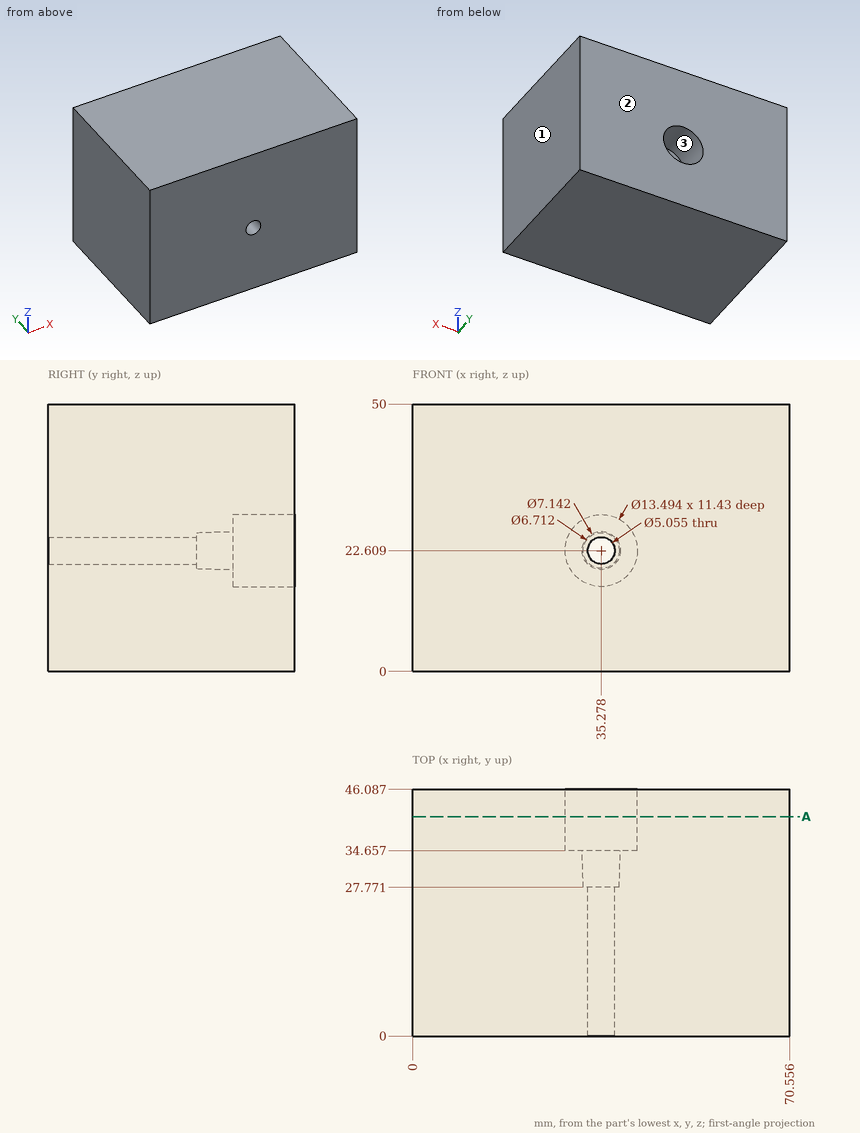
Job drawing, mm, ordinate dimensions from the low corner. One solid piece. Give positions to 0.01 mm unless a question says otherwise; leave off trailing zeros. Write each loop counter-clockwise with the first axis right and the second up, starting at its lowest first coordinate (ties: lowest second). Pieces come first, ordered by that corner, then holes. Notation, with made-up numbers: M 8,79.25 L 22,79.25 A7 ccw 22,90.25 Z; hole C 13.25,2.5 d6. An arc over 180 degrees is marked long. One line per item, written item: value. Start each with the question number.
Q1. Drop a flat-ended pin along its axis: pin 1 Ø6.5 at (x, z) = (35, 25) entering from +Y. Give the stop position or say it passes through.
Q2. Two-plate mould, pull along X, no slides. Class the marked faces 1, 2 and 3: +X half, -X half, draft (parallel to the pull), parting line (faces both ways), or undercut.
Q3. Saw through at A-A, the plane y = 41. Write the cut outline in (x, z) (1 decimal), plus the area to 4 significant figures.
Q4. Probe probe 1 along Z at (x, y) = (35.5, 3); probe 2 along X at (y, z) = (7, 24) (1 decimal). List the from-to ranges inside material, lowest first. Write a range as [from, to].
Output values:
1. pin 1: stops at y = 34.66
2. face 1: +X half
2. face 2: draft
2. face 3: undercut
3. outline: M 0,0 L 70.6,0 L 70.6,50 L 0,50 Z; hole C 35.3,22.6 d13.5
3. area: 3,385 mm²
4. probe 1: z = [0, 20.09], [25.13, 50]
4. probe 2: x = [0, 33.2], [37.4, 70.6]
